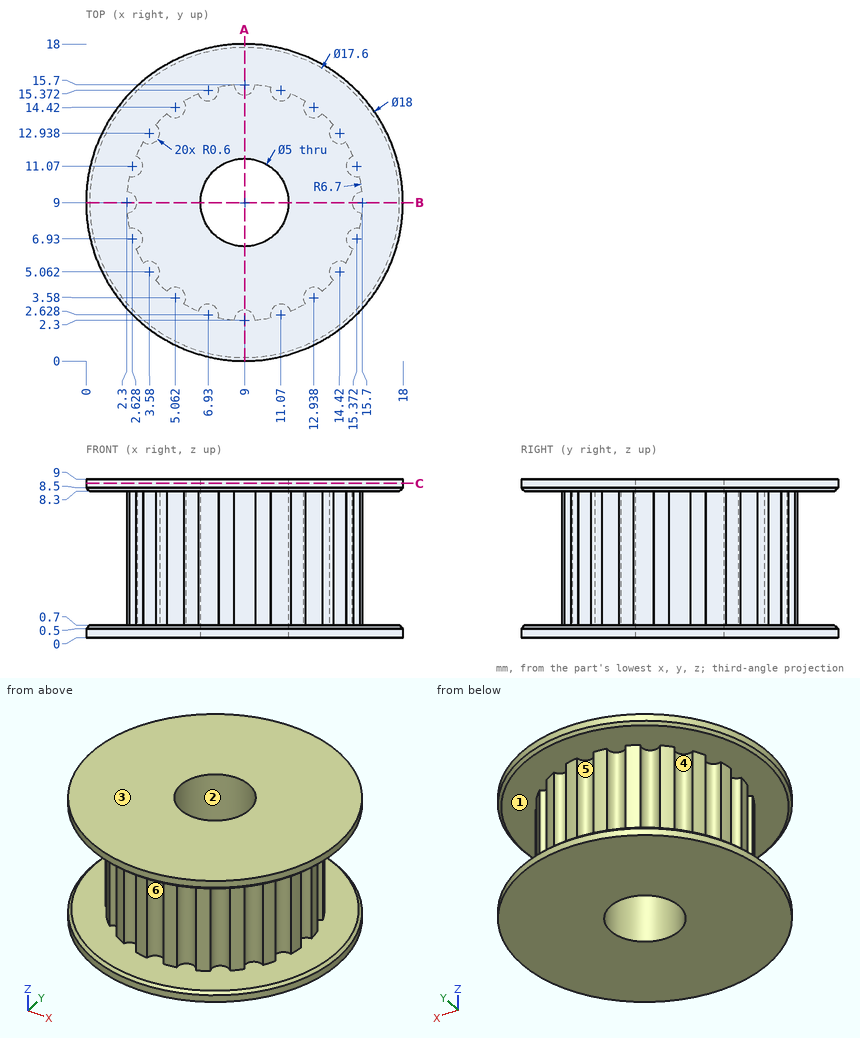
Source: three-view drawing plus pictorial views. Frame: mm from the lowest corner of the part. A direction names the side the tool comes from. Coordinates: 2 decimals unless noted, no trailing zeros. Order: outer loops, then holes, each group sorted by start corner. A loop starts at its lowest first (then second) coordinate and runs counter-clockwise, first axis right, second up.
Item 1: Material intervals for line 1 (Z direction, x = 13.5, y = 14.75); line 2 (X direction, y = 13, z = 5), sorted ascending.
Output values:
line 1: z = 0 to 0.7, 8.3 to 9
line 2: x = 4.18 to 13.82
Item 2: First-contact query: P1, Ø1, axis at x = 3, y = 10.5, coming from the -Z side. Flat tip, straight axial feed; report the tip coordinate or a pass-through.
Output values:
P1: stops at z = 0
Item 3: Cut plane A-A (x = 9). Return loops of the section in (y, z).
Output values:
outline: (0, 0) - (6.5, 0) - (6.5, 9) - (0, 9) - (0, 8.5) - (0.2, 8.3) - (2.9, 8.3) - (2.9, 0.7) - (0.2, 0.7) - (0, 0.5) - close; (11.5, 0) - (18, 0) - (18, 0.5) - (17.8, 0.7) - (15.1, 0.7) - (15.1, 8.3) - (17.8, 8.3) - (18, 8.5) - (18, 9) - (11.5, 9) - close
Item 4: Pull-direction query (Z, two-part tool) for the marked faces 1, 2 and 3; classes: pulls with the +Z half, pulls with the -Z half, needs draft (parallel to the pull), parting line crosses it, or undercut.
Output values:
face 1: undercut
face 2: needs draft
face 3: pulls with the +Z half
Item 5: Cut plane C-C (z = 8.75). Return loops of the section in (x, y).
Output values:
outline: circle Ø18 at (9, 9); hole circle Ø5 at (9, 9)
Item 6: Set-up query: the marked faces 4, 5 and 6. Return all of +Z, -Z, +X, -X, +Y, -Y with unobstructed straight access to the full face (end or side cutting, diameter ignored); none if empty.
Output values:
face 4: none
face 5: +Y
face 6: -Y
